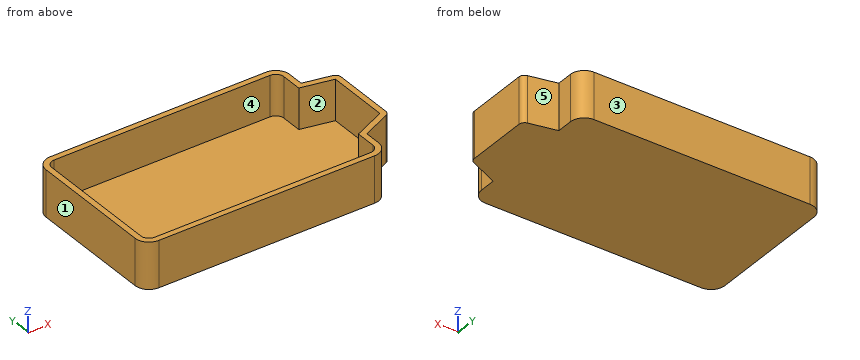
```python
from build123d import *

# Parameters (mm, degrees)
EXTRUDE_DEPTH    = 40
EXTRUDE001_DEPTH = 40


with BuildPart() as extrude_body:
    # Sketch → Extrude (new body)
    with BuildSketch(Plane.XY):
        with BuildLine():
            Line((-92.929424, 60.081154), (93.998491, 60.081154))
            ThreePointArc((100.998491, 53.081154), (98.948238, 58.030901), (93.998491, 60.081154))
            Line((100.998491, 53.081154), (100.998491, 35.048241))
            Line((100.998491, 35.048241), (128.657806, 29.335068))
            Line((128.657806, 29.335068), (128.657806, -24.680387))
            Line((128.657806, -24.680387), (100.998491, -37.405182))
            Line((100.998491, -37.405182), (100.998491, -54.803909))
            ThreePointArc((93.998491, -61.803909), (98.948238, -59.753656), (100.998491, -54.803909))
            Line((93.998491, -61.803909), (-92.929424, -61.803909))
            ThreePointArc((-99.929424, -54.803909), (-97.879172, -59.753656), (-92.929424, -61.803909))
            Line((-99.929424, -54.803909), (-99.929424, 53.081154))
            ThreePointArc((-92.929424, 60.081154), (-97.879172, 58.030901), (-99.929424, 53.081154))
        make_face()
    extrude(amount=EXTRUDE_DEPTH)


with BuildPart() as extrude_body_1:
    # Extrude placement: moved
    add(extrude_body.part.moved(Location((0, 0, 5))))


with BuildPart() as bottom:
    # Offset2D → Extrude001 (new body)
    with BuildSketch(Plane(origin=(14.364191, -0.861378, 0), x_dir=(0, 1, 0), z_dir=(0, 0, 1))):
        with BuildLine():
            Line((53.942531, 119.293615), (-53.942531, 119.293615))
            ThreePointArc((-53.942531, 119.293615), (-62.427812, 115.778897), (-65.942531, 107.293615))
            Line((-65.942531, 107.293615), (-65.942531, -79.6343))
            ThreePointArc((-65.942531, -79.6343), (-62.427812, -88.119581), (-53.942531, -91.6343))
            Line((-53.942531, -91.6343), (-39.74728, -91.6343))
            Line((-39.74728, -91.6343), (-28.361368, -116.383348))
            ThreePointArc((-28.361368, -116.383348), (-26.516354, -118.503643), (-23.819009, -119.293615))
            Line((-23.819009, -119.293615), (30.196446, -119.293615))
            ThreePointArc((30.196446, -119.293615), (33.354204, -118.170284), (35.093079, -115.30504))
            Line((35.093079, -115.30504), (39.982392, -91.6343))
            Line((39.982392, -91.6343), (53.942531, -91.6343))
            ThreePointArc((53.942531, -91.6343), (62.427812, -88.119581), (65.942531, -79.6343))
            Line((65.942531, -79.6343), (65.942531, 107.293615))
            ThreePointArc((65.942531, 107.293615), (62.427812, 115.778897), (53.942531, 119.293615))
        make_face()
    extrude(amount=EXTRUDE001_DEPTH)

    # Cut: cut Extrude body
    add(extrude_body_1.part, mode=Mode.SUBTRACT)


solid = bottom.part
```
Geometry: final body of the model. Coordinates: model frame, mm. Face numbers are marked on the shaded views. A direction names the side the tool comes from. Coordinates: 2 decimals unless noted, no trailing zeros. Order: outer loops, then holes, each group sorted by start corner. A loop starts at its lowest first (then second) coordinate and runs counter-clockwise, first axis right, second up. Notation, with made-up numbers: (17, 23) -> (28, 23) arc R23 cw to (28, 57) -> close; hole circle Ø8 at (40, 72.25). An arc over 180 degrees is marked (long way). Answer in a Markdown table with one row per item.
Item 1: Access query for the marked faces 4 and 5. Directions: +Z, -Z, +X, -X, +Y, -Y. A direction counts if a zero-diameter tool reaches every point of the face in a straight line with its end or side. Return the directions, or none.
Return value:
| item | result |
|---|---|
| face 4 | +Z |
| face 5 | +Z, -Z, +X, +Y |
Item 2: Section A-A on z = 13.5. Output: boundary loops of the cut face in (x, y), plus the area to 3 significant figures.
Return value:
| item | result |
|---|---|
| outline | (-104.93, -54.8) arc R12 ccw to (-92.93, -66.8) -> (94, -66.8) arc R12 ccw to (106, -54.8) -> (106, -40.61) -> (130.75, -29.22) arc R5 ccw to (133.66, -24.68) -> (133.66, 29.34) arc R5 ccw to (129.67, 34.23) -> (106, 39.12) -> (106, 53.08) arc R12 ccw to (94, 65.08) -> (-92.93, 65.08) arc R12 ccw to (-104.93, 53.08) -> close; hole (-99.93, -54.8) arc R7 ccw to (-92.93, -61.8) -> (94, -61.8) arc R7 ccw to (101, -54.8) -> (101, -37.41) -> (128.66, -24.68) -> (128.66, 29.34) -> (101, 35.05) -> (101, 53.08) arc R7 ccw to (94, 60.08) -> (-92.93, 60.08) arc R7 ccw to (-99.93, 53.08) -> close |
| area | 3,440 mm² |
Item 3: Ray query, L1, parallel to Y at x = 43, z = 25; L2, parallel to X at y = 22, z = 23.5; L3, parallel to X at y = -51, z = 6.5. Return the intervals inside material, ascending.
Return value:
| item | result |
|---|---|
| L1 | y = -66.8 to -61.8, 60.08 to 65.08 |
| L2 | x = -104.93 to -99.93, 128.66 to 133.66 |
| L3 | x = -104.93 to -99.93, 101 to 106 |
Item 4: Contact query for flat-ended pins moving along their axis: P1, Ø4.5, axis at y = -49.5, z = 21.5, coming from the +X side; P2, Ø3, axis at x = 109.5, z = 13.5, coming from the -Y side; P3, Ø10, axis at x = 48, y = 46, coming from the +Z side. Output: stop coordinate, or through.
Return value:
| item | result |
|---|---|
| P1 | stops at x = 106 |
| P2 | stops at y = -39.69 |
| P3 | stops at z = 5 |
Item 5: Section B-B on x = 86. Output: boundary loops of the cut face in (y, z).
Return value:
| item | result |
|---|---|
| outline | (-66.8, 0) -> (65.08, 0) -> (65.08, 40) -> (60.08, 40) -> (60.08, 5) -> (-61.8, 5) -> (-61.8, 40) -> (-66.8, 40) -> close |
Item 6: Section C-C on y = -45. Output: boundary loops of the cut face in (x, z).
Return value:
| item | result |
|---|---|
| outline | (-104.93, 0) -> (106, 0) -> (106, 40) -> (101, 40) -> (101, 5) -> (-99.93, 5) -> (-99.93, 40) -> (-104.93, 40) -> close |
Item 7: Draft query along Y for the marked faces 1, 2 and 3. Return one class per face: released by +Y, released by -Y, zero draft, split by the parting line, or undercut.
Return value:
| item | result |
|---|---|
| face 1 | zero draft |
| face 2 | undercut |
| face 3 | released by +Y |
